Check sheet for the modelled part. Datum: model origin and axes. Units: mm. Give positions to 0.01 mm unless a question says otherwise; leave off trailing zeros. Order: outer loops, then holes, each group sorted by start corner. A loop starts at its lowest first (then second) coordinate and runs counter-clockwise, first axis right, second up. Notation, with made-up numbers: (81, 3.5) -> (139, 3.5) arc R22 cw to (139, 35.5) -> close; hole circle Ø10 at (-24.75, -15). An arc over 180 degrees is marked (long way). Answer in a Markdown table with one row per item. Add a question column.
(1) Cross-section at D-D (x = 16.5). Record the cut outline in (y, z).
(2) Thickness scan on L1, parallel to X at y = 19.5, z = 0.85; L2, parallel to Y at x = 1, z = 1.05; L3, parallel to Y at x = 7, z = 1.25. Record the ranges inside material, lowest first. Write a range as [from, to].
(3) Cross-section at C-C (x = 5). Record the cut outline in (y, z).
(4) Go/stop test with flat-tipped pins: pin 1 (0.7 mm diameter, centred on x = 19, z = 1, fed in from +Y); pin 2 (0.5 mm diameter, centred on y = -40, z = 1, fed in from +X). Record where each tip stops, or that it passes through.
(5) Cross-section at A-A (y = 9). Record the cut outline in (x, z).
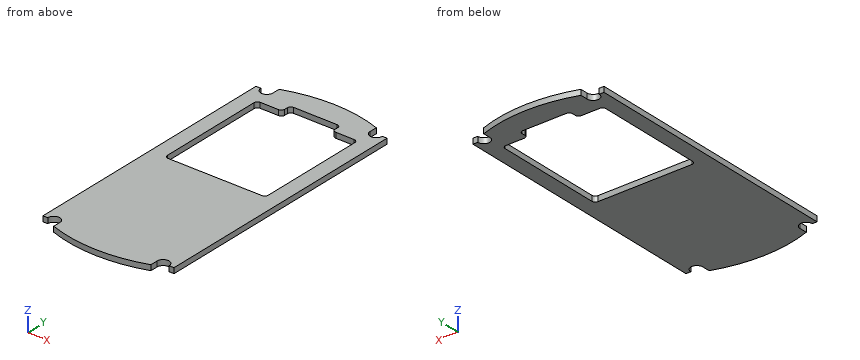
```python
from build123d import *

# Parameters (mm, degrees)
EXTRUDE_1_DEPTH     = 1.6
CUT_EXTRUDE_1_DEPTH = 10
FILLET_2_R          = 1


with BuildPart() as part:
    # 草图1 → 凸台-拉伸1 (new body)
    with BuildSketch(Plane.XY):
        with BuildLine():
            Line((-19.5, 0), (-19.5, 39.264880132))
            Line((-19.5, 39.264880132), (-18.064045876, 39.264880132))
            ThreePointArc((-18.064045876, 39.264880132), (-16.264045876, 37.464880132), (-14.464045876, 39.264880132))
            Line((-14.464045876, 39.264880132), (-14.464045876, 41.554679362))
            ThreePointArc((-14.464045876, 41.554679362), (0, 44), (14.464045876, 41.554679362))
            Line((14.464045876, 41.554679362), (14.464045876, 39.264880132))
            ThreePointArc((14.464045876, 39.264880132), (16.264045876, 37.464880132), (18.064045876, 39.264880132))
            Line((18.064045876, 39.264880132), (19.5, 39.264880132))
            Line((19.5, 39.264880132), (19.5, 0))
            Line((19.5, 0), (19.5, -39.264880132))
            Line((19.5, -39.264880132), (18.064045876, -39.264880132))
            ThreePointArc((18.064045876, -39.264880132), (16.264045876, -37.464880132), (14.464045876, -39.264880132))
            Line((14.464045876, -39.264880132), (14.464045876, -41.554679362))
            ThreePointArc((14.464045876, -41.554679362), (0, -44), (-14.464045876, -41.554679362))
            Line((-14.464045876, -41.554679362), (-14.464045876, -39.264880132))
            ThreePointArc((-14.464045876, -39.264880132), (-16.264045876, -37.464880132), (-18.064045876, -39.264880132))
            Line((-18.064045876, -39.264880132), (-19.5, -39.264880132))
            Line((-19.5, -39.264880132), (-19.5, 0))
        make_face()
    extrude(amount=EXTRUDE_1_DEPTH)

    # 草图2 → 切除-拉伸1 (cut)
    with BuildSketch(Plane.XY.offset(1.6)):
        Polygon((-15, 0), (15, 0), (15, 34), (7.5, 34), (7.5, 37), (-7.5, 37), (-7.5, 34), (-15, 34), align=None)
    extrude(amount=-CUT_EXTRUDE_1_DEPTH, mode=Mode.SUBTRACT)

    # 圆角2
    fillet_2_edges = [part.edges().sort_by_distance(p)[0] for p in [
        (7.5, 37, 0.8),
        (7.5, 34, 0.8),
        (15, 34, 0.8),
        (15, 0, 0.8),
        (-15, 0, 0.8),
        (-15, 34, 0.8),
        (-7.5, 34, 0.8),
        (-7.5, 37, 0.8),
    ]]
    fillet(fillet_2_edges, radius=FILLET_2_R)


solid = part.part
```
Answer below:
| question | item | result |
|---|---|---|
| 1 | outline | (-37.48, 0) -> (37.48, 0) -> (37.48, 1.6) -> (-37.48, 1.6) -> close |
| 2 | L1 | x = [-19.5, -15], [15, 19.5] |
| 2 | L2 | y = [-43.99, 0], [37, 43.99] |
| 2 | L3 | y = [-43.44, 0], [36.87, 43.44] |
| 3 | outline | (-43.71, 0) -> (0, 0) -> (0, 1.6) -> (-43.71, 1.6) -> close; (37, 0) -> (43.71, 0) -> (43.71, 1.6) -> (37, 1.6) -> close |
| 4 | pin 1 | stops at y = 39.26 |
| 4 | pin 2 | stops at x = 14.46 |
| 5 | outline | (-19.5, 0) -> (-15, 0) -> (-15, 1.6) -> (-19.5, 1.6) -> close; (15, 0) -> (19.5, 0) -> (19.5, 1.6) -> (15, 1.6) -> close |
